Source: CAD feature listing. Evaluate the final solid. Frame: model axes, mm. Coordinates: 2 decimals unless noted, no trailing zeros. Loops run counter-clockwise (first coordinate to the right, second up) from the corner with the lowest first, then second, coordinate; pieces in that order, holes last. Notation, with made-up numbers: (80.5, -2.5) - (132.5, -2.5) arc R19 ccw to (132.5, 20.5) - close; hole circle Ø1 at (5, 28). An arc over 180 degrees is marked (long way). Use CSV: the item, a comma, the result in double quotes. Start each with the question number.
```python
from build123d import *

# Parameters (mm, degrees)
SKETCH2_R               = 13.335
SKETCH2_R_2             = 10.287
BOSS_EXTRUDE2_DEPTH     = 87
CUT_EXTRUDE1_DEPTH      = 20
CUT_EXTRUDE1_DEPTH_BACK = 20
SKETCH4_R               = 2.6


with BuildPart() as part:
    # Sketch2 → Boss-Extrude2 (new body)
    with BuildSketch(Plane(origin=(0, 0, 0), x_dir=(1, 0, 0), z_dir=(0, 1, 0))):
        with Locations(Location((0, 0, 0), (0, 0, 270))):
            Circle(SKETCH2_R)
        with Locations(Location((0, 0, 0), (0, 0, 270))):
            Circle(SKETCH2_R_2, mode=Mode.SUBTRACT)
    extrude(amount=BOSS_EXTRUDE2_DEPTH)

    # Sketch4 → Cut-Extrude1 (cut, two sides: drawn at the far end of the back side and taken through both)
    with BuildSketch(Plane(origin=(-1275.101492903, -824.70990816, -345.604288183), x_dir=(-0.965175873824897, 0, -0.2616018589122535), z_dir=(0.2616018589122535, 2.2232920799531116e-15, -0.965175873824897)).offset(-CUT_EXTRUDE1_DEPTH_BACK)):
        with Locations(Location((-1321.107921864, 901.70990816, 0), (0, 0, 180))):
            Circle(SKETCH4_R)
        with Locations(Location((-1321.107921864, 836.70990816, 0), (0, 0, 180))):
            Circle(SKETCH4_R)
    extrude(amount=CUT_EXTRUDE1_DEPTH + CUT_EXTRUDE1_DEPTH_BACK, mode=Mode.SUBTRACT)


solid = part.part
```
(1) Draft query along X for faces 1 (the cylindrical face through (9.01, 42.89, -9.83)), 2 (the cylindrical face through (6.952, 42.891, -7.582)), 3 (the flat face through (-8, 0, 7)). Return one class per face: released by +X, released by -X, zero draft, split by the parting line, or undercut.
(2) Section C-C on y = 44.5. Output: boundary loops of the cut face in (x, z) (3 decimals), plus the area to 3 significant figures.
(3) Section B-B on x = 8.5. Output: boundary loops of the cut face in (y, z).
(4) Ray query, line 1 (X direction, y = 40.5, z = 0) (3 decimals); line 2 (Y direction, x = 2.5, z = -11.5); line 3 (Z direction, x = 8.75, y = 14). Return the intervals inside material, ascending. Write a range as [from, to].
(5) Section A-A on z = 0. Output: boundary loops of the cut face in (x, y) (3 decimals).
(6) Pin query (flat end, axial travel): pin 1 Ø8 at (x, z) = (-10.5, 1) entering from -Y; pin 2 Ø2 at (x, y) = (-1.5, 27.5) entering from -Z; pin 3 Ø1.5 at (y, z) = (10, -10) entering from -X. Return the tip coordinate at first contact, or that it passes through.
(7) Section D-D on x = -4.5. State how many separate pieces and enclosed holes the cut face has, plus the area to 3 significant figures.
Solution:
1,face 1,"split by the parting line"
1,face 2,"undercut"
1,face 3,"zero draft"
2,outline,"circle Ø26.67 at (0, 0); hole circle Ø20.574 at (0, 0)"
2,area,"226 mm²"
3,outline,"(0, -10.27) - (87, -10.27) - (87, -5.79) - (0, -5.79) - close; (0, 5.79) - (87, 5.79) - (87, 10.27) - (0, 10.27) - close"
4,line 1,"x = [-13.335, -10.287], [10.287, 13.335]"
4,line 2,"y = [0, 9.47], [14.53, 74.47], [79.53, 87]"
4,line 3,"z = [-10.06, -5.41], [5.41, 10.06]"
5,outline,"(-13.335, 0) - (-10.287, 0) - (-10.287, 87) - (-13.335, 87) - close; (10.287, 0) - (13.335, 0) - (13.335, 87) - (10.287, 87) - close"
6,pin 1,"stops at y = 0"
6,pin 2,"stops at z = -13.33"
6,pin 3,"stops at x = -9.61"
7,separate pieces,"4"
7,enclosed holes,"0"
7,area,"547 mm²"
